Check sheet for the modelled part. Datum: model origin and axes. Units: mm. A direction names the side the tool comes from. Give positions to 0.01 mm unless a question says otherwise; leave off trailing zeros. Order: outer loops, then holes, each group sorted by start corner. A loop starts at its lowest first (then second) coordinate and runs counter-clockwise, first axis right, second up.
```python
from build123d import *

# Parameters (mm, degrees)
SKETCH_1_W          = 47
SKETCH_1_H          = 5
EXTRUDE_1_DEPTH     = 19
SKETCH_2_R          = 23.5
EXTRUDE_2_DEPTH     = 5
SKETCH_3_R          = 6
SKETCH_3_R_2        = 1.5
CUT_EXTRUDE_1_DEPTH = 5
M2_5X0_45_1_D       = 2.05
M2_5X0_45_1_DEPTH   = 7.25
M2_5X0_45_1_TIP     = 0.615882135
CUT_EXTRUDE_2_DEPTH = 5
CUT_EXTRUDE_3_DEPTH = 5


with BuildPart() as part:
    # ｽｹｯﾁ1 → ﾎﾞｽ - 押し出し1 (new body)
    with BuildSketch(Plane.XY):
        Rectangle(SKETCH_1_W, SKETCH_1_H)
    extrude(amount=EXTRUDE_1_DEPTH)

    # ｽｹｯﾁ2 → ﾎﾞｽ - 押し出し2 (add)
    with BuildSketch(Plane.XZ.offset(2.5)):
        with Locations((0, 19)):
            Circle(SKETCH_2_R)
    extrude(amount=-EXTRUDE_2_DEPTH)

    # ｽｹｯﾁ3 → ｶｯﾄ - 押し出し1 (cut)
    with BuildSketch(Plane.XZ.offset(2.5)):
        with Locations(Location((0, 26, 0), (0, 0, 270))):  # turned: the seam where the file's is
            Circle(SKETCH_3_R)
        with Locations(Location((-15.5, 19, 0), (0, 0, 270))):  # turned: the seam where the file's is
            Circle(SKETCH_3_R_2)
        with Locations(Location((7.75, 5.576606241, 0), (0, 0, 270))):  # turned: the seam where the file's is
            Circle(SKETCH_3_R_2)
        with Locations(Location((7.75, 32.423393759, 0), (0, 0, 270))):  # turned: the seam where the file's is
            Circle(SKETCH_3_R_2)
    extrude(amount=-CUT_EXTRUDE_1_DEPTH, mode=Mode.SUBTRACT)

    # M2.5x0.45 ねじ穴1
    with Locations(Plane(origin=(0, 0, 0), x_dir=(-1, 0, 0), z_dir=(0, 0, -1))):
        with Locations((18, 0), (-18, 0)):
            Hole(M2_5X0_45_1_D / 2, depth=M2_5X0_45_1_DEPTH)
            with Locations((0, 0, -(M2_5X0_45_1_DEPTH + M2_5X0_45_1_TIP / 2))):  # 118° drill point
                Cone(0, M2_5X0_45_1_D / 2, M2_5X0_45_1_TIP, mode=Mode.SUBTRACT)

    # ｽｹｯﾁ8 → ｶｯﾄ - 押し出し2 (cut)
    with BuildSketch(Plane(origin=(0, 2.5, 0), x_dir=(1, 0, 0), z_dir=(0, 1, 0))):
        with BuildLine():
            Line((-13.829316686, 0), (13.829316686, 0))
            ThreePointArc((13.829316686, 0), (0, 4.5), (-13.829316686, 0))
        make_face()
    extrude(amount=-CUT_EXTRUDE_2_DEPTH, mode=Mode.SUBTRACT)

    # ｽｹｯﾁ9 → ｶｯﾄ - 押し出し3 (cut)
    with BuildSketch(Plane(origin=(0, 2.5, 0), x_dir=(1, 0, 0), z_dir=(0, 1, 0))):
        with BuildLine():
            Line((-10, -40.266170318), (10, -40.266170318))
            ThreePointArc((10, -40.266170318), (0, -42.5), (-10, -40.266170318))
        make_face()
    extrude(amount=-CUT_EXTRUDE_3_DEPTH, mode=Mode.SUBTRACT)


solid = part.part
```
Q1. Sectioned sample at B-B, the plane x = 7.75. Record the cut outline in (y, z), plus the area to 3 significant figures.
Q2. Sectioned sample at D-D, the plane z = 22.5. Record the cut outline in (x, y).
Q3. Draft check along X on faces 1 (the cylindrical face through (-19.74, -0.04, 31.75)), 2 (the conical face through (18.13, 0.12, 7.76)), 3 (the flat face through (0, 0, 0)), 4 (the cylindrical face through (19.939, -0.035, 31.437)). Enter one of: pulls with the +X half, pulls with the -X half, needs draft (parallel to the pull), parting line crosses it, or undercut.
Q4. Tool access check on faces 5 (the flat face through (0, 2.5, 16)), 6 (the cylindrical face through (-19.024, 0.045, 3.676)). Record the directions out of +Z, -Z, +X, -X, +Y, -Y that give a thin tool (end or side, any length) a straight path to the whole face; none if there is none.
Q5. Sectioned sample at C-C, the plane x = 0. Record the cut outline in (y, z).
Q6. Sectioned sample at A-A, the plane z = 5.5. Record the cut outline in (x, y) (3 decimals), plus the area to 3 significant figures.
Q7. Material ranges on line 1 (X direction, y = -0.35, z = 19); line 2 (X direction, y = 0, z = 4.5) (3 decimals); line 3 (X direction, y = 1.4, z = 26), recorded low to high.
Q8. Go/stop test with flat-tipped pins: P1, Ø2.5, axis at x = -18, y = 0, coming from the +Z side; P2, Ø2.5, axis at x = 7.75, z = 32.42, coming from the -Y side; P3, Ø1.6, axis at x = 18, y = 0, coming from the -Z side. Record where each tip stops, or that it passes through.
Filled in:
1. outline: (-2.5, 0) - (2.5, 0) - (2.5, 4.08) - (-2.5, 4.08) - close; (-2.5, 7.08) - (2.5, 7.08) - (2.5, 30.92) - (-2.5, 30.92) - close; (-2.5, 33.92) - (2.5, 33.92) - (2.5, 40.27) - (-2.5, 40.27) - close
1. area: 171 mm2
2. outline: (-23.24, -2.5) - (-4.87, -2.5) - (-4.87, 2.5) - (-23.24, 2.5) - close; (4.87, -2.5) - (23.24, -2.5) - (23.24, 2.5) - (4.87, 2.5) - close
3. face 1: pulls with the -X half
3. face 2: undercut
3. face 3: needs draft
3. face 4: pulls with the +X half
4. face 5: +Z, -Z, +X, -X, +Y
4. face 6: -Z
5. outline: (-2.5, 0) - (2.5, 0) - (2.5, 20) - (-2.5, 20) - close; (-2.5, 32) - (2.5, 32) - (2.5, 40.27) - (-2.5, 40.27) - close
6. outline: (-23.5, -2.5) - (6.252, -2.5) - (6.252, 2.5) - (-23.5, 2.5) - close; (9.248, -2.5) - (23.5, -2.5) - (23.5, 2.5) - (9.248, 2.5) - close; hole circle Ø2.05 at (-18, 0); hole circle Ø2.05 at (18, 0)
6. area: 213 mm2
7. line 1: x = -23.5 to -17, -14 to 23.5
7. line 2: x = -23.5 to -19.025, -16.975 to 6.706, 8.794 to 16.975, 19.025 to 23.5
7. line 3: x = -22.43 to -6, 6 to 22.43
8. P1: stops at z = 35.48
8. P2: passes through
8. P3: stops at z = 7.39
